from build123d import *

# Parameters (mm, degrees)
F0_R      = 53.975
F1_DEPTH  = 25.4
F2_R      = 50.8
F3_DEPTH  = 19.05
F4_R      = 9.525
F5_DEPTH  = 6.35
F6_W      = 17.119241
F6_H      = 19.05
F7_DEPTH  = 6.35
F8_R      = 7.9375
F9_DEPTH  = 6.35
F11_DEPTH = 3.175


with BuildPart() as f1:
    # F0 (on Top) → F1 (new body)
    with BuildSketch(Plane.XY):
        Circle(F0_R)
    extrude(amount=F1_DEPTH)

    # F2 (on face) → F3 (cut)
    with BuildSketch(Plane(origin=(0, 0, 0), x_dir=(1, 0, 0), z_dir=(0, 0, -1))):
        Circle(F2_R)
    extrude(amount=-F3_DEPTH, mode=Mode.SUBTRACT)

    # F4 (on face) → F5 (cut, through all)
    with BuildSketch(Plane.XY.offset(25.4)):
        with Locations((41.91, 0)):
            Circle(F4_R)
    extrude(amount=-F5_DEPTH, mode=Mode.SUBTRACT)

    # F6 (on face) → F7 (cut, through all)
    with BuildSketch(Plane.XY.offset(25.4)):
        with Locations((50.46962, 0)):
            Rectangle(F6_W, F6_H)
    extrude(amount=-F7_DEPTH, mode=Mode.SUBTRACT)

    # F8 (on face) → F9 (cut, through all)
    with BuildSketch(Plane.XY.offset(25.4)):
        Circle(F8_R)
    extrude(amount=-F9_DEPTH, mode=Mode.SUBTRACT)

    # F10 (on face) → F11 (cut)
    with BuildSketch(Plane.XY.offset(25.4)):
        with BuildLine():
            ThreePointArc((0, -15.875), (1.122532, -15.410032), (1.5875, -14.2875))
            Line((1.5875, -14.2875), (1.5875, 14.2875))
            ThreePointArc((1.5875, 14.2875), (1.122532, 15.410032), (0, 15.875))
            ThreePointArc((0, 15.875), (-1.122532, 15.410032), (-1.5875, 14.2875))
            Line((-1.5875, 14.2875), (-1.5875, -14.2875))
            ThreePointArc((-1.5875, -14.2875), (-1.122532, -15.410032), (0, -15.875))
        make_face()
    extrude(amount=-F11_DEPTH, mode=Mode.SUBTRACT)


solid = f1.part
Input: part model. Units: mm. Frame: model coordinates. A direction names the side the tool comes from. Give positions to 0.01 mm unless a question says otherwise; leave off trailing zeros. Order: outer loops, then holes, each group sorted by start corner. A loop starts at its lowest first (then second) coordinate and runs counter-clockwise, first axis right, second up. Notation, with made-up numbers: (15, 78) -> (41, 78) arc R24 cw to (41, 113) -> close; hole circle Ø2 at (39.25, -3.5). An arc over 180 degrees is marked (long way). Use one line per item in the form item = value.
1) Line query: probe 1 along Y at (x, z) = (0, 21) (1 decimal); probe 2 along Y at (x, z) = (0, 6.75) (3 decimals); probe 3 along Z at (x, y) = (-11, -8). Output: solid intervals per line, ascending.
Response values:
probe_1 = -54 to -7.9, 7.9 to 54
probe_2 = -53.975 to -50.8, 50.8 to 53.975
probe_3 = 19.05 to 25.4
2) Reachability of faces 1 (the flat face through (52, 0, 19.05)), 2 (the cylindrical face through (-11.012, 49.592, 9.392)), 3 (the flat face through (-1.588, -11, 24)) from +Z, -Z, +X, -X, +Y, -Y: full face, straight path, thin tool, end or side. Return the list, or none.
Response values:
face_1 = +Z, +X
face_2 = -Z
face_3 = +Z
3) Section A-A, the plane y = 0. Count the separate pieces of the cut face and the enclosed holes in it, and give its area (3 significant figures).
Response values:
separate_pieces = 3
enclosed_holes = 0
area = 569 mm^2
4) Mould query, pull axis Y, two halves, no side actions, for faces 4 (the flat face through (40, -32, 0)), 5 (the cylindrical face through (32.387, 0.209, 22.269)), 6 (the cylindrical face through (-39.78, 36.48, 12.52)). Classes: pulls with the +Y half, pulls with the -Y half, needs draft (parallel to the pull), parting line crosses it, or undercut.
Response values:
face_4 = needs draft
face_5 = undercut
face_6 = parting line crosses it
5) First-contact query: pin 1 Ø2 at (x, y) = (-37, 25.5) entering from -Z; pin 2 Ø1.6 at (x, y) = (0, 13) entering from +Z (3 decimals); pin 3 Ø4 at (x, z) = (13.5, 19.5) entering from -Y. Flat tips, straight axial feed; report the tip coordinate or a pass-through.
Response values:
pin_1 = 19.05
pin_2 = 22.225
pin_3 = -52.74
6) Section C-C, the plane x = -36. Return loops of the section in (y, z).
Response values:
outline = (-40.22, 0) -> (-35.84, 0) -> (-35.84, 19.05) -> (35.84, 19.05) -> (35.84, 0) -> (40.22, 0) -> (40.22, 25.4) -> (-40.22, 25.4) -> close
